```python
from build123d import *

# Parameters (mm, degrees)
BOSS_EXTRUDE1_DEPTH = 3.175
SKETCH2_W           = 89.027
SKETCH2_H           = 78.74
BOSS_EXTRUDE2_DEPTH = 6.35
CUT_EXTRUDE1_DEPTH  = 3.175
SKETCH4_W           = 89.027
SKETCH4_H           = 78.74
BOSS_EXTRUDE3_DEPTH = 3.175


with BuildPart() as part:
    # Sketch1 → Boss-Extrude1 (new body)
    with BuildSketch(Plane(origin=(0, 0, 0), x_dir=(1, 0, 0), z_dir=(0, 1, 0))):
        with BuildLine():
            Line((2.54, 0), (80.01, 0))
            ThreePointArc((80.01, 0), (81.806051224, 0.743948776), (82.55, 2.54))
            Line((82.55, 2.54), (82.55, 69.596))
            ThreePointArc((82.55, 69.596), (81.806051224, 71.392051224), (80.01, 72.136))
            Line((80.01, 72.136), (2.54, 72.136))
            ThreePointArc((2.54, 72.136), (0.743948776, 71.392051224), (0, 69.596))
            Line((0, 69.596), (0, 2.54))
            ThreePointArc((0, 2.54), (0.743948776, 0.743948776), (2.54, 0))
        make_face()
    extrude(amount=BOSS_EXTRUDE1_DEPTH)

    # Sketch2 → Boss-Extrude2 (add)
    with BuildSketch(Plane(origin=(0, 3.175, 0), x_dir=(1, 0, 0), z_dir=(0, 1, 0))):
        with Locations((41.275, 36.068)):
            Rectangle(SKETCH2_W, SKETCH2_H)
    extrude(amount=BOSS_EXTRUDE2_DEPTH)

    # Sketch3 → Cut-Extrude1 (cut)
    with BuildSketch(Plane(origin=(0, 9.525, 0), x_dir=(1, 0, 0), z_dir=(0, 1, 0))):
        with BuildLine():
            Line((6.731, 8.128), (63.246, 8.128))
            ThreePointArc((63.246, 8.128), (66.421, 4.953), (69.596, 8.128))
            Line((69.596, 8.128), (75.819, 8.128))
            Line((75.819, 8.128), (75.819, 64.008))
            Line((75.819, 64.008), (59.944, 64.008))
            ThreePointArc((59.944, 64.008), (56.769, 67.183), (53.594, 64.008))
            Line((53.594, 64.008), (6.731, 64.008))
            Line((6.731, 64.008), (6.731, 8.128))
        make_face()
    extrude(amount=-CUT_EXTRUDE1_DEPTH, mode=Mode.SUBTRACT)

    # Sketch4 → Boss-Extrude3 (add)
    with BuildSketch(Plane(origin=(0, 9.525, 0), x_dir=(1, 0, 0), z_dir=(0, 1, 0))):
        with Locations((41.275, 36.068)):
            Rectangle(SKETCH4_W, SKETCH4_H)
        with BuildLine():
            Line((6.731, 11.43), (1.524, 11.43))
            Line((1.524, 11.43), (1.524, 60.706))
            Line((1.524, 60.706), (6.731, 60.706))
            Line((6.731, 60.706), (6.731, 64.008))
            Line((6.731, 64.008), (53.594, 64.008))
            ThreePointArc((53.594, 64.008), (56.769, 67.183), (59.944, 64.008))
            Line((59.944, 64.008), (75.819, 64.008))
            Line((75.819, 64.008), (75.819, 60.706))
            Line((75.819, 60.706), (81.026, 60.706))
            Line((81.026, 60.706), (81.026, 11.43))
            Line((81.026, 11.43), (75.819, 11.43))
            Line((75.819, 11.43), (75.819, 8.128))
            Line((75.819, 8.128), (69.596, 8.128))
            ThreePointArc((69.596, 8.128), (66.421, 4.953), (63.246, 8.128))
            Line((63.246, 8.128), (6.731, 8.128))
            Line((6.731, 8.128), (6.731, 11.43))
        make_face(mode=Mode.SUBTRACT)
    extrude(amount=BOSS_EXTRUDE3_DEPTH)


solid = part.part
```
Source: CAD feature listing. Evaluate the final solid. Frame: model axes, mm. A direction names the side the tool comes from. Round coordinates to 2 decimals unless told otherwise and drop trailing zeros. Loops run counter-clockwise (first coordinate to the right, second up) from the corner with the lowest first, then second, coordinate; pieces in that order, holes last. Notation, with made-up numbers: (62.5, 8.25) - (100.5, 8.25) arc R17 cw to (100.5, 30.25) - close; hole circle Ø11 at (40.5, 26.5). An arc over 180 degrees is marked (long way). Use CSV: the item, a comma, the result in double quotes.
Q1. Mould query, pull axis X, two halves, no side actions, for faces 4 (the flat face through (75.819, 8, -36)), 5 (the flat face through (38, 3.175, 2)), 6 (the cylindrical face through (0.724, 1.565, -0.764)). Classes: pulls with the +X half, pulls with the -X half, needs draft (parallel to the pull), parting line crosses it, or undercut.
Reported:
face 4,"undercut"
face 5,"needs draft"
face 6,"pulls with the -X half"
Q2. Ray query, line 1 along Z through (x, y) = (52, 11.5); line 2 along X through (y, z) = (10, -24.5); line 3 along Y through (x, z) = (47, -44.5). Return the intervals inside material, ascending.
Reported:
line 1,"-75.44 to -64.01, -8.13 to 3.3"
line 2,"-3.24 to 1.52, 81.03 to 85.79"
line 3,"0 to 6.35"
Q3. Reachability of faces 1 (the flat face through (81.026, 11, -36)), 2 (the flat face through (42, 2, -72.136)), 3 (the flat face through (82.55, 2, -36)) from +Z, -Z, +X, -X, +Y, -Y: full face, straight path, thin tool, end or side. Return the list, or none.
Reported:
face 1,"+Y"
face 2,"-Z, +X, -X, -Y"
face 3,"+Z, -Z, +X, -Y"
Q4. Section query C-C, the plane x = 39.5. Output: boundary loops of the cut face in (y, z) (3 decimals).
Reported:
outline,"(0, -72.136) - (3.175, -72.136) - (3.175, -75.438) - (12.7, -75.438) - (12.7, -64.008) - (6.35, -64.008) - (6.35, -8.128) - (12.7, -8.128) - (12.7, 3.302) - (3.175, 3.302) - (3.175, 0) - (0, 0) - close"
Q5. Pin query (flat end, axial travel): pin 1 Ø3 at (x, z) = (24, -53) entering from +Y; pin 2 Ø1.6 at (x, y) = (53.5, 1) entering from -Z; pin 3 Ø5.5 at (x, z) = (5, -48.5) entering from +Y (3 decimals). Return the tip coordinate at first contact, or that it passes through.
Reported:
pin 1,"y = 6.35"
pin 2,"z = -72.14"
pin 3,"y = 9.525"
Q6. Section query D-D, the plane x = 66. Output: boundary loops of the cut face in (y, z) (3 decimals).
Reported:
outline,"(0, -72.136) - (3.175, -72.136) - (3.175, -75.438) - (12.7, -75.438) - (12.7, -64.008) - (6.35, -64.008) - (6.35, -4.981) - (12.7, -4.981) - (12.7, 3.302) - (3.175, 3.302) - (3.175, 0) - (0, 0) - close"
